```python
from build123d import *

# Parameters (mm, degrees)
BOSS_EXTRUDE1_DEPTH       = 90
BOSS_EXTRUDE2_DEPTH       = 1
SKETCH3_W                 = 50
SKETCH3_H                 = 60
BOSS_EXTRUDE3_DEPTH       = 8
FILLET1_R                 = 20
FILLET1_R_2               = 8
F_8_CLEARANCE_HOLE1_D     = 4.4958
F_8_CLEARANCE_HOLE1_DEPTH = 15
F_8_CLEARANCE_HOLE1_TIP   = 1.350674586
SKETCH8_R                 = 3.5
CUT_EXTRUDE2_DEPTH        = 12.7
CUT_EXTRUDE1_DEPTH        = 6
FILLET2_R                 = 10
FILLET3_R                 = 2


# Some blends are built 0.0001 mm under size
with BuildPart() as part:
    # Sketch1 → Boss-Extrude1 (new body)
    with BuildSketch(Plane(origin=(0, 0, 0), x_dir=(1, 0, 0), z_dir=(0, 1, 0))):
        with BuildLine():
            Line((-15, -5), (-15, 5))
            ThreePointArc((-15, 5), (0, 20), (15, 5))
            Line((15, 5), (15, -5))
            ThreePointArc((15, -5), (0, -20), (-15, -5))
        make_face()
    extrude(amount=BOSS_EXTRUDE1_DEPTH)

    # Sketch2 → Boss-Extrude2 (add)
    with BuildSketch(Plane.XZ):
        with BuildLine():
            Line((-21, 5), (-21, -5))
            ThreePointArc((-21, -5), (0, -26), (21, -5))
            Line((21, -5), (21, 5))
            ThreePointArc((21, 5), (0, 26), (-21, 5))
        make_face()
    extrude(amount=BOSS_EXTRUDE2_DEPTH)

    # Sketch3 → Boss-Extrude3 (add)
    with BuildSketch(Plane(origin=(0, 90, 0), x_dir=(1, 0, 0), z_dir=(0, 1, 0))):
        Rectangle(SKETCH3_W, SKETCH3_H)
    extrude(amount=BOSS_EXTRUDE3_DEPTH)

    # Fillet1
    # the kernel refuses this fillet: 20, 8 mm, written as the material it adds along each edge
    with BuildSketch(Plane(origin=(0, 0, 5), x_dir=(1, 0, 0), z_dir=(0, 0, -1))) as fillet1_piece_1:
        with BuildLine():
            CenterArc((35, -14.282856857), FILLET1_R, 134.427004001, 45.572995999)
            Line((21, 0), (20.72, 0.285657137))
            ThreePointArc((20.72, 0.285657137), (18, 0.4), (15, 0.4))
            Line((15, 0.4), (14.6, 0))
            Line((14.6, 0), (14.6, -14.282856857))
            Line((14.6, -14.282856857), (15, -14.282856857))
        make_face()
    revolve(axis=Axis((0, 0, 5), (0, -1, 0)), revolution_arc=180)
    with BuildSketch(Plane(origin=(0, 90, 5), x_dir=(1, 0, 0), z_dir=(0, 0, -1))) as fillet1_piece_2:
        with BuildLine():
            CenterArc((15 + FILLET1_R_2, FILLET1_R_2), FILLET1_R_2, 180, 90)
            Line((15, FILLET1_R_2), (15 - FILLET1_R_2 * 0.02, FILLET1_R_2))
            Line((15 - FILLET1_R_2 * 0.02, FILLET1_R_2), (15 - FILLET1_R_2 * 0.02, -FILLET1_R_2 * 0.02))
            Line((15 - FILLET1_R_2 * 0.02, -FILLET1_R_2 * 0.02), (15 + FILLET1_R_2, -FILLET1_R_2 * 0.02))
            Line((15 + FILLET1_R_2, -FILLET1_R_2 * 0.02), (15 + FILLET1_R_2, 0))
        make_face()
    revolve(axis=Axis((0, 90, 5), (0, -1, 0)), revolution_arc=180)
    with BuildSketch(Plane(origin=(15, 90, -5), x_dir=(1, 0, 0), z_dir=(0, 0, 1)), Plane(origin=(-15, 90, 5), x_dir=(-1, 0, 0), z_dir=(0, 0, -1))) as fillet1_piece_3:
        with BuildLine():
            CenterArc((FILLET1_R_2, -FILLET1_R_2), FILLET1_R_2, 90, 90)
            Line((0, -FILLET1_R_2), (-FILLET1_R_2 * 0.02, -FILLET1_R_2))
            Line((-FILLET1_R_2 * 0.02, -FILLET1_R_2), (-FILLET1_R_2 * 0.02, FILLET1_R_2 * 0.02))
            Line((-FILLET1_R_2 * 0.02, FILLET1_R_2 * 0.02), (FILLET1_R_2, FILLET1_R_2 * 0.02))
            Line((FILLET1_R_2, FILLET1_R_2 * 0.02), (FILLET1_R_2, 0))
        make_face()
    extrude(amount=10)
    with BuildSketch(Plane(origin=(0, 90, -5), x_dir=(-1, 0, 0), z_dir=(0, 0, 1))) as fillet1_piece_4:
        with BuildLine():
            CenterArc((15 + FILLET1_R_2, FILLET1_R_2), FILLET1_R_2, 180, 90)
            Line((15, FILLET1_R_2), (15 - FILLET1_R_2 * 0.02, FILLET1_R_2))
            Line((15 - FILLET1_R_2 * 0.02, FILLET1_R_2), (15 - FILLET1_R_2 * 0.02, -FILLET1_R_2 * 0.02))
            Line((15 - FILLET1_R_2 * 0.02, -FILLET1_R_2 * 0.02), (15 + FILLET1_R_2, -FILLET1_R_2 * 0.02))
            Line((15 + FILLET1_R_2, -FILLET1_R_2 * 0.02), (15 + FILLET1_R_2, 0))
        make_face()
    revolve(axis=Axis((0, 90, -5), (0, -1, 0)), revolution_arc=180)
    with BuildSketch(Plane(origin=(15, 0, -5), x_dir=(0, 1, 0), z_dir=(0, 0, 1)), Plane(origin=(-15, 0, 5), x_dir=(0, 1, 0), z_dir=(0, 0, -1))) as fillet1_piece_5:
        with BuildLine():
            CenterArc((14.282856857, -20), FILLET1_R, 90, 45.572995999)
            Line((0, -6), (-0.285657137, -5.72))
            ThreePointArc((-0.285657137, -5.72), (-0.4, -3), (-0.4, 0))
            Line((-0.4, 0), (0, 0.4))
            Line((0, 0.4), (14.282856857, 0.4))
            Line((14.282856857, 0.4), (14.282856857, 0))
        make_face()
    extrude(amount=10)
    with BuildSketch(Plane(origin=(0, 0, -5), x_dir=(-1, 0, 0), z_dir=(0, 0, 1))) as fillet1_piece_6:
        with BuildLine():
            CenterArc((35, -14.282856857), FILLET1_R, 134.427004001, 45.572995999)
            Line((21, 0), (20.72, 0.285657137))
            ThreePointArc((20.72, 0.285657137), (18, 0.4), (15, 0.4))
            Line((15, 0.4), (14.6, 0))
            Line((14.6, 0), (14.6, -14.282856857))
            Line((14.6, -14.282856857), (15, -14.282856857))
        make_face()
    revolve(axis=Axis((0, 0, -5), (0, -1, 0)), revolution_arc=180)

    # #8 Clearance Hole1
    with Locations(Plane(origin=(0, 98, 0), x_dir=(1, 0, 0), z_dir=(0, 1, 0))):
        with Locations((-18, 23), (18, 23), (18, -23), (-18, -23)):
            Hole(F_8_CLEARANCE_HOLE1_D / 2, depth=F_8_CLEARANCE_HOLE1_DEPTH)
            with Locations((0, 0, -(F_8_CLEARANCE_HOLE1_DEPTH + F_8_CLEARANCE_HOLE1_TIP / 2))):  # 118° drill point
                Cone(0, F_8_CLEARANCE_HOLE1_D / 2, F_8_CLEARANCE_HOLE1_TIP, mode=Mode.SUBTRACT)

    # Sketch8 → Cut-Extrude2 (cut)
    with BuildSketch(Plane.XZ.offset(1)):
        with Locations(Location((0, 0, 0), (0, 0, 270))):
            Circle(SKETCH8_R)
    extrude(amount=-CUT_EXTRUDE2_DEPTH, mode=Mode.SUBTRACT)

    # Sketch7 → Cut-Extrude1 (cut)
    with BuildSketch(Plane.XZ.offset(1)):
        Polygon((-3.464101615, -6), (3.464101615, -6), (6.92820323, 0), (3.464101615, 6), (-3.464101615, 6), (-6.92820323, 0), align=None)
    extrude(amount=-CUT_EXTRUDE1_DEPTH, mode=Mode.SUBTRACT)

    # Fillet2
    fillet2_edges = [part.edges().sort_by_distance(p)[0] for p in [
        (-25, 94, -30),
        (-25, 94, 30),
        (25, 94, 30),
        (25, 94, -30),
    ]]
    fillet(fillet2_edges, radius=FILLET2_R)

    # Fillet3
    fillet3_edges = [part.edges().sort_by_distance(p)[0] for p in [
        (0, 90, 30),
        (-25, 90, 0),
        (0, 90, -30),
        (25, 90, 0),
        (22.071067812, 90, 27.071067812),
        (22.071067812, 90, -27.071067812),
        (-22.071067812, 90, -27.071067812),
        (-22.071067812, 90, 27.071067812),
    ]]
    fillet(fillet3_edges, radius=FILLET3_R - 0.0001)  # a hair under: the kernel refuses the full size


solid = part.part
```
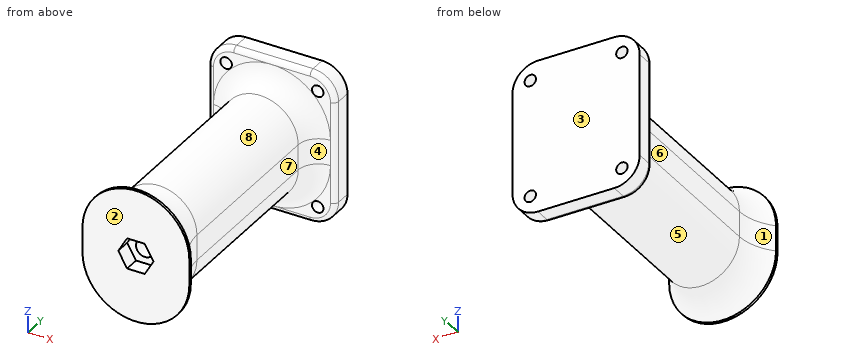
Here's how the part is built. I have some questions about the finished solid (model axes, mm). Face numbers are marked on the shaded views. A direction names the side the tool comes from. Round coordinates to 2 decimals unless told otherwise and drop trailing zeros. Loops run counter-clockwise (first coordinate to the right, second up) from the corner with the lowest first, then second, coordinate; pieces in that order, holes last.
1. Will these pins go through, and if not, where does the flat tip stop? pin 1 (0.5 mm diameter, centred on y = -0.5, z = -1.5, fed in from +X); pin 2 (1.8 mm diameter, centred on x = 1, y = 3.5, fed in from -Z); pin 3 (6 mm diameter, centred on x = 0.5, z = -0.5, fed in from -Y).
Answers:
pin 1: stops at x = 21
pin 2: stops at z = -23.74
pin 3: stops at y = 5
2. Thinking about a two-plate mould opening in Y: for the marked faces 1, 2, 3 and 4, which applies, released by +Y, released by -Y, zero draft, split by the parting line, or undercut?
Answers:
face 1: undercut
face 2: released by -Y
face 3: released by +Y
face 4: undercut
3. Suppose I cut it at B-B, the plane y = 9. Please give me the cut outline in (x, z).
Answers:
outline: (-15.71, -5) arc R15.71 ccw to (15.71, -5) - (15.71, 5) arc R15.71 ccw to (-15.71, 5) - close; hole circle Ø7 at (0, 0)
4. For the marked faces 5, 6, 7 and 8, which set-ups out of +Z, -Z, +X, -X, +Y, -Y let a thin tool reach every point of the face, with its end or its side?
Answers:
face 5: -Z
face 6: +Z, -Z, -X
face 7: +Z, -Z, +X
face 8: +Z
5. If I drill on probe 1 along X at (y, z) = (95.5, -23); probe 2 along Y at (x, z) = (-17.5, -20); probe 3 along X at (y, z) = (9, 0), over which ranges is the centre line in solid material (lowest first)?
Answers:
probe 1: x = -24.54 to -20.25, -15.75 to 15.75, 20.25 to 24.54
probe 2: y = 90 to 98
probe 3: x = -15.71 to -3.5, 3.5 to 15.71
6. Suppose I cut it at C-C, the plane y = 33. Please give me the cut outline in (x, z), and give its area (3 significant figures).
Answers:
outline: (-15, -5) arc R15 ccw to (15, -5) - (15, 5) arc R15 ccw to (-15, 5) - close
area: 1,010 mm2
7. Suppose I cut it at D-D, the plane z = -23. Give the number of separate pieces and of enclosed holes in the cut face, and give its area (3 significant figures).
Answers:
separate pieces: 4
enclosed holes: 0
area: 416 mm2
